from build123d import *


with BuildPart() as f1:
    # F0 (on Front) → F1 (revolve)
    with BuildSketch(Plane.XZ):
        with BuildLine():
            Line((-6.858, 0), (0, 0))
            Line((0, 0), (0, 68.58))
            Line((0, 68.58), (-0.1016, 68.58))
            ThreePointArc((-0.1016, 68.58), (-4.412123, 66.794523), (-6.1976, 62.484))
            Line((-6.1976, 62.484), (-6.1976, 8.370646))
            ThreePointArc((-6.1976, 8.370646), (-6.514543, 7.531252), (-7.307179, 7.110819))
            ThreePointArc((-7.307179, 7.110819), (-9.526559, 5.933606), (-10.414, 3.583302))
            Line((-10.414, 3.583302), (-10.414, 3.556))
            ThreePointArc((-10.414, 3.556), (-9.372472, 1.041528), (-6.858, 0))
        make_face()
    revolve(axis=Axis((0, 0, 34.29), (0, 0, -1)))


solid = f1.part
Source: CAD feature listing. Evaluate the final solid. Frame: model axes, mm. A direction names the side the tool comes from. Give positions to 0.01 mm unless a question says otherwise; leave off trailing zeros. Write each loop counter-clockwise with the first axis right and the second up, starting at its lowest first coordinate (ties: lowest second). Pieces come first, ordered by that corner, then holes. Notation, with made-up numbers: (45, 23) -> (53, 23) arc R23 cw to (53, 61) -> close; hole circle Ø11 at (-35, 26.25). An arc over 180 degrees is marked (long way). Return JSON: item names as keys, results as strings. Group by question number.
1. Access query for faces 1 (the face through (-5.725, -2.374, 35.049)), 2 (the face through (0, 0, 0)). Directions: +Z, -Z, +X, -X, +Y, -Y. A direction counts if a zero-diameter tool reaches every point of the face in a straight line with its end or side. Return the directions, or none.
2. Section A-A, the plane z = 13. Output: boundary loops of the cut face in (x, y).
3. Material intervals for line 1 (X direction, y = -0.75, z = 41); line 2 (Z direction, x = 8.25, y = -0.75); line 3 (Z direction, x = -8, y = -5.5), sorted ascending. Write a range as from..to.
4. Pin query (flat end, axial travel): pin 1 Ø12 at (y, z) = (2, 55) entering from -X; pin 2 Ø1 at (x, z) = (2.5, 25) entering from +Y; pin 3 Ø1.5 at (y, z) = (-2, 35) entering from +X. Return the tip coordinate at first contact, or that it passes through.
Determined:
{
 "1": {"face 1": "+Z", "face 2": "-Z, +X, -X, +Y, -Y"},
 "2": {"outline": "circle Ø12.4 at (0, 0)"},
 "3": {"line 1": "x = -6.15..6.15", "line 2": "z = 0.3..6.84", "line 3": "z = 1.43..5.71"},
 "4": {"pin 1": "stops at x = -6.2", "pin 2": "stops at y = 5.87", "pin 3": "stops at x = 6.07"}
}
